```python
from build123d import *

# Parameters (mm, degrees)
EXTRUDE_1_DEPTH     = 150
EXTRUDE_START       = -247.5
EXTRUDE_2_DEPTH     = 247.5
SKETCH_3_R          = 52.6
CUT_EXTRUDE_1_DEPTH = 52.5
SKETCH_4_R          = 52.6
CUT_EXTRUDE_2_DEPTH = 82.5
SKETCH_6_R          = 1.5
CUT_EXTRUDE_3_DEPTH = 165
SKETCH_7_R          = 1.5
CUT_EXTRUDE_4_DEPTH = 165
CUT_EXTRUDE_5_DEPTH = 500
CUT_EXTRUDE_START   = -53
SKETCH_9_R          = 52.6
CUT_EXTRUDE_6_DEPTH = 53


with BuildPart() as part:
    # 草图1 → 凸台-拉伸1 (new, symmetric)
    with BuildSketch(Plane.XY):
        with BuildLine():
            Line((-52.413174316, -16.669107897), (-49.363680538, -15.699268892))
            ThreePointArc((-49.363680538, -15.699268892), (-16.314268086, -49.163855187), (30.185108172, -42.096309157))
            Line((30.185108172, -42.096309157), (32.049825279, -44.696853352))
            ThreePointArc((32.049825279, -44.696853352), (-17.322099319, -52.201004542), (-52.413174316, -16.669107897))
        make_face()
    extrude(amount=EXTRUDE_1_DEPTH, both=True)

    # 草图2 → 凸台-拉伸2 (add)
    with BuildSketch(Plane(origin=(0, 0, -150), x_dir=(-1, 0, 0), z_dir=(0, 0, -1)).offset(EXTRUDE_START)):
        with BuildLine():
            Line((-24.924043095, -42.002946324), (-23.507517235, -46.158819671))
            ThreePointArc((-23.507517235, -46.158819671), (-34.198599667, -38.906243468), (-42.762509098, -29.233676054))
            Line((-42.762509098, -29.233676054), (-40.120809695, -27.427734676))
            ThreePointArc((-40.120809695, -27.427734676), (-33.774000748, -34.946772003), (-26.042778843, -41.033323898))
            ThreePointArc((-26.042778843, -41.033323898), (-25.447325167, -41.476499857), (-24.924043095, -42.002946324))
        make_face()
        with BuildLine():
            Line((48.558861257, 1.99924822), (51.756152533, 2.130885963))
            ThreePointArc((51.756152533, 2.130885963), (50.673816706, -10.742639362), (46.439539695, -22.947966205))
            Line((46.439539695, -22.947966205), (45.090508335, -18.769695848))
            ThreePointArc((45.090508335, -18.769695848), (45.195249795, -18.034849445), (45.40762753, -17.323607076))
            ThreePointArc((45.40762753, -17.323607076), (47.966326083, -7.822503569), (48.558861257, 1.99924822))
        make_face()
    extrude(amount=EXTRUDE_2_DEPTH)

    # 草图3 → 切除-拉伸1 (cut)
    with BuildSketch(Plane(origin=(0, 0, -150), x_dir=(-1, 0, 0), z_dir=(0, 0, -1))):
        Circle(SKETCH_3_R)
    extrude(amount=-CUT_EXTRUDE_1_DEPTH, mode=Mode.SUBTRACT)

    # 草图4 → 切除-拉伸2 (cut, symmetric)
    with BuildSketch(Plane.XY):
        Circle(SKETCH_4_R)
    extrude(amount=CUT_EXTRUDE_2_DEPTH, both=True, mode=Mode.SUBTRACT)

    # 草图6 → 切除-拉伸3 (cut)
    with BuildSketch(Plane(origin=(0, 0, 0), x_dir=(-0.6991347993064156, -0.7149898827247683, 0), z_dir=(0.7149898827247683, -0.6991347993064156, 0))):
        with Locations((0, 90)):
            Circle(SKETCH_6_R)
        with Locations((0, -90)):
            Circle(SKETCH_6_R)
    extrude(amount=CUT_EXTRUDE_3_DEPTH, mode=Mode.SUBTRACT)

    # 草图7 → 切除-拉伸4 (cut)
    with BuildSketch(Plane(origin=(0, 0, 0), x_dir=(0.13298935431462466, -0.991117466115384, 0), z_dir=(0.991117466115384, 0.13298935431462466, 0))):
        with Locations(Location((0, 90, 0), (0, 0, 180))):
            Circle(SKETCH_7_R)
        with Locations(Location((0, -90, 0), (0, 0, 180))):
            Circle(SKETCH_7_R)
    extrude(amount=-CUT_EXTRUDE_4_DEPTH, mode=Mode.SUBTRACT)

    # 草图8 → 切除-拉伸5 (cut)
    with BuildSketch(Plane(origin=(0, 0, -150), x_dir=(-1, 0, 0), z_dir=(0, 0, -1))):
        with BuildLine():
            Line((-24.924043095, -42.002946324), (-23.132074518, -47.240524219))
            ThreePointArc((-23.132074518, -47.240524219), (16.570504001, -49.921722698), (46.789382897, -24.031513647))
            Line((46.789382897, -24.031513647), (45.090508335, -18.769695848))
            Line((45.090508335, -18.769695848), (-24.924043095, -42.002946324))
        make_face()
    extrude(amount=-CUT_EXTRUDE_5_DEPTH, mode=Mode.SUBTRACT)

    # 草图9 → 切除-拉伸6 (cut)
    with BuildSketch(Plane.XY.offset(150).offset(CUT_EXTRUDE_START)):
        Circle(SKETCH_9_R)
    extrude(amount=CUT_EXTRUDE_6_DEPTH, mode=Mode.SUBTRACT)


solid = part.part
```
Geometry: final body of the model. Coordinates: model frame, mm. A direction names the side the tool comes from. Coordinates: 2 decimals unless noted, no trailing zeros. Order: outer loops, then holes, each group sorted by start corner. A loop starts at its lowest first (then second) coordinate and runs counter-clockwise, first axis right, second up. Notation, with made-up numbers: M 38,8.5 L 56,8.5 A18 ccw 56,42.5 Z; hole C 14,41 d1. An arc over 180 degrees is marked long. Answer in a Markdown table with one row per item. Add a question column.
Q1. Section query B-B on x = 0. Return the cut outline in (y, z).
Q2. Section query D-D on z = 7.5. Return the cut outline in (x, y).
Q3. Reachability of faces 5 (the cylindrical face through (33.873, -34.851, -91.562)), 6 (the flat face through (-49, -11, -82.5)), 7 (the flat face through (33, -38, 82.5)), 8 (the cylindrical face through (-51.357, -6.763, 88.24)), 9 (the flat face through (-49, -11, 97)) from +Z, -Z, +X, -X, +Y, -Y: full face, straight path, thin tool, end or side. Return the list, or none.
Q4. Section query C-C on y = -1.5. Return the cut outline in (x, z), and give its area (3 significant figures).
Q5. Line query: L1, parallel to Y at x = 1, z = -100; L2, parallel to X at y = -45, z = 127.5; L3, parallel to Y at x = -16, z = 53. Output: solid intervals per line, ascending.
Q6. Mould query, pull axis Z, two halves, no side actions, for faces 1 (the cylindrical face through (-16.632, -52.425, 2.1)), 2 (the flat face through (33, -37, -97.5)), 3 (the flat face through (-49, -11, 82.5)), 4 (the flat face through (33, -38, 97)). Classes: released by +Z, released by -Z, zero draft, split by the parting line, or undercut.
Q7. Section query A-A on y = -50. Return the cut outline in (x, z), and give its area (3 significant figures).
Q8. Contact query for flat-ended pins moving along their axis: P1, Ø10, axis at x = 34.5, y = -38.5, coming from the +Z side; P2, Ø12, axis at x = 14, z = 114.5, coming from the +Y side; P3, Ø21.5, axis at x = 31, y = -32.5, coming from the -Z side; P4, Ø10, axis at x = 35, y = -36.5, coming from the -Z side. Output: stop coordinate, or through.
Completed:
| question | item | result |
|---|---|---|
| 1 | outline | M -55,-150 L -52.6,-150 L -52.6,150 L -55,150 Z |
| 2 | outline | M -52.41,-16.67 A55 ccw 32.05,-44.7 L 30.65,-42.75 A52.6 cw -50.13,-15.94 Z |
| 3 | face 5 | +Z, -Z, +Y |
| 3 | face 6 | +X, +Y |
| 3 | face 7 | +Y |
| 3 | face 8 | +Z, -Z, -X |
| 3 | face 9 | +Z, +X, +Y |
| 4 | outline | M -51.78,-97.5 L -48.58,-97.5 L -48.58,-82.5 L -51.78,-82.5 Z; M -51.78,82.5 L -48.58,82.5 L -48.58,97 L -51.78,97 Z |
| 4 | area | 94.4 mm2 |
| 5 | L1 | y = -54.99 to -52.59 |
| 5 | L2 | x = -31.62 to -27.24, 27.24 to 31.62 |
| 5 | L3 | y = -52.62 to -50.11 |
| 6 | face 1 | zero draft |
| 6 | face 2 | released by -Z |
| 6 | face 3 | undercut |
| 6 | face 4 | released by +Z |
| 7 | outline | M -22.91,-150 L -16.33,-150 L -16.33,150 L -22.91,150 Z; M 16.33,-150 L 22.91,-150 L 22.91,150 L 16.33,150 Z |
| 7 | area | 3,950 mm2 |
| 8 | P1 | stops at z = 97 |
| 8 | P2 | stops at y = -48.65 |
| 8 | P3 | stops at z = -150 |
| 8 | P4 | stops at z = -97.5 |
